Geometry: see drawing. Coordinates: mm, zero at the bounding-box minimum. A direction names the side the tool comes from. Give positions to 0.01 mm unless a question says otherwise; leave off trailing zeros. Write each loop counter-clockwise with the first axis right and the second up, starting at its lowest first coordinate (ties: lowest second). Pieces come first, ordered by that corner, then holes. Notation, with made-up numbers: (-4.5, -34.75) - (52.5, -34.75) arc R12 cw to (52.5, -16.75) - close; hole circle Ø5 at (-30.5, -1). An arc over 180 degrees is marked (long way). Use CSV: the item, a comma, the result in double quotes. Start each with the question number.
(1) Section C-C on z = 4. Output: boundary loops of the cut face in (x, y), and give its area (3 significant figures).
(2) Line query: probe 1 along Y at (x, z) = (5.25, 45); probe 2 along Z at (x, y) = (5, 5.75); probe 3 along X at (y, z) = (5.5, 35.5). Output: solid intervals per line, ascending. Write a range as [from, to].
(3) Section A-A on y = 5.25. Output: boundary loops of the cut face in (x, z), and give its area (3 significant figures).
(4) First-contact query: pin 1 Ø1 at (x, y) = (6.5, 6) entering from +Z; pin 2 Ø6 at (y, z) = (5.5, 12.5) entering from -X; pin 3 Ø2 at (x, y) = (4.5, 6) entering from -Z; pin 4 Ø5 at (y, z) = (2.5, 33.5) entering from +X. Flat tips, straight axial feed; report the tip coordinate or a pass-through.
(5) Section D-D on x = 2.5. Output: boundary loops of the cut face in (y, z), and give its area (3 significant figures).
(6) Reachability of the marked faces 1, 2 and 3 from +Z, -Z, +X, -X, +Y, -Y: full face, straight path, thin tool, end or side. Return the list, or none.
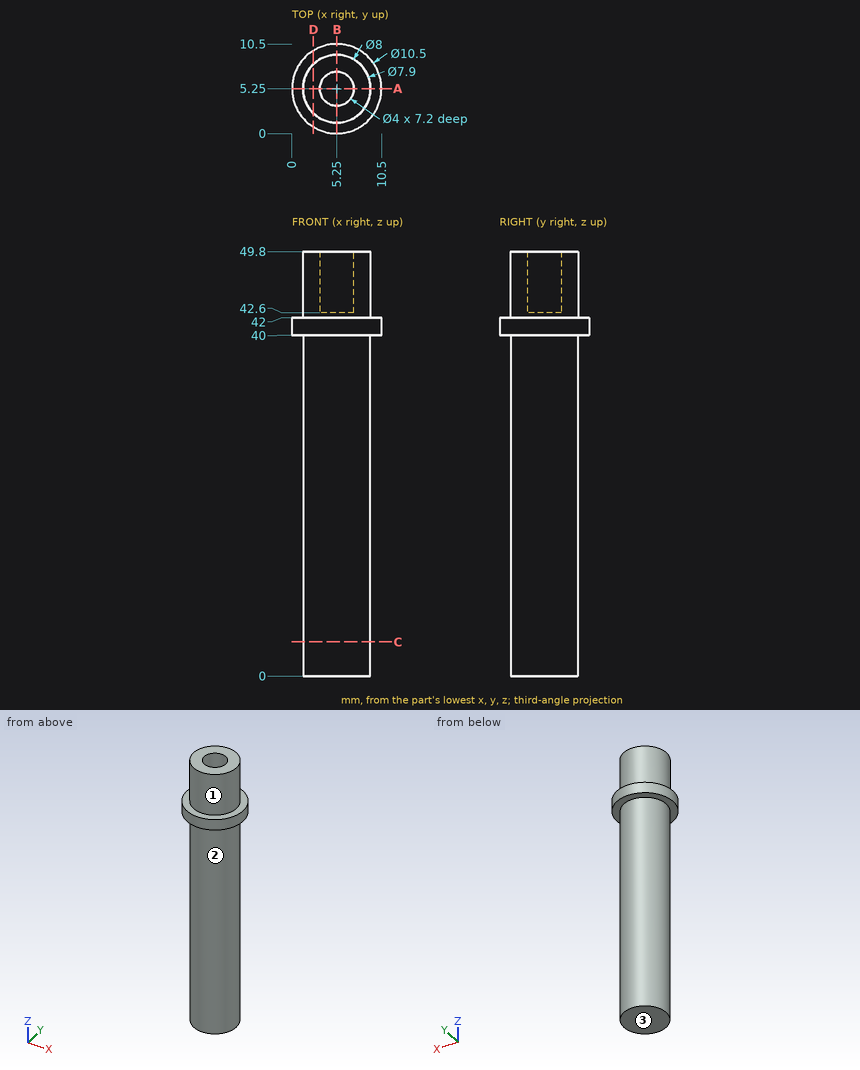
Check values:
1,outline,"circle Ø7.9 at (5.25, 5.25)"
1,area,"49.0 mm²"
2,probe 1,"y = [1.25, 3.25], [7.25, 9.25]"
2,probe 2,"z = [0, 42.6]"
2,probe 3,"x = [1.31, 9.19]"
3,outline,"(0, 40) - (1.3, 40) - (1.3, 0) - (9.2, 0) - (9.2, 40) - (10.5, 40) - (10.5, 42) - (9.25, 42) - (9.25, 49.8) - (7.25, 49.8) - (7.25, 42.6) - (3.25, 42.6) - (3.25, 49.8) - (1.25, 49.8) - (1.25, 42) - (0, 42) - close"
3,area,"371 mm²"
4,pin 1,"stops at z = 42.6"
4,pin 2,"stops at x = 1.3"
4,pin 3,"stops at z = 0"
4,pin 4,"stops at x = 9.19"
5,outline,"(0.78, 40) - (2.41, 40) - (2.41, 0) - (8.09, 0) - (8.09, 40) - (9.72, 40) - (9.72, 42) - (8.15, 42) - (8.15, 49.8) - (2.35, 49.8) - (2.35, 42) - (0.78, 42) - close"
5,area,"290 mm²"
6,face 1,"+Z"
6,face 2,"-Z"
6,face 3,"-Z, +X, -X, +Y, -Y"
